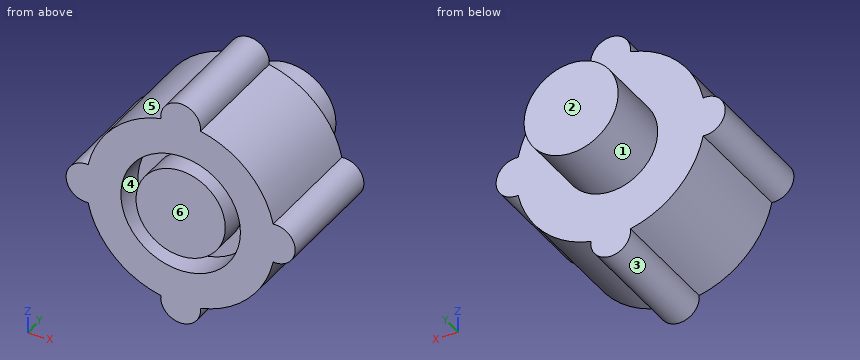
Autodesk Inventor part; units mm, degrees
ref_plane "YZ Plane" through (0, 0, 0) normal (1, 0, 0) x (0, 1, 0)
ref_plane "XZ Plane" through (0, 0, 0) normal (0, 1, 0) x (-1, 0, 0)
ref_plane "XY Plane" through (0, 0, 0) normal (0, 0, 1) x (1, 0, 0)
sketch "Sketch1" plane through (0, 0, 0) normal (0, 1, 0) x (-1, 0, 0)
  circle A0 centre (0, 0) radius 9.5
  dimension "d0" = 19
extrude "Extrusion1" add sketch "Sketch1" along normal blind 12
sketch "Sketch2" plane through (0, 12, 0) normal (0, 1, 0) x (1, 0, 0)
  circle A0 centre (0, 0) radius 4.7244
  dimension "d9" = 9.4488
extrude "Extrusion2" add sketch "Sketch2" along normal blind 6.9088
sketch "Sketch3" plane through (0, 0, 0) normal (0, -1, 0) x (1, 0, 0)
  circle A0 centre (0, 0) radius 4.48
  circle A1 centre (0, 0) radius 6
  dimension "d5" = 12
  dimension "d6" = 1.52
extrude "Extrusion3" cut sketch "Sketch3" against normal blind 3
sketch "Sketch4" plane through (0, 12, 0) normal (0, 1, 0) x (1, 0, 0)
  circle A0 centre (0, 0) radius 9.5
  circle A1 centre (-9.5, 0) radius 2
  line L0 (-15.7, 0) -> (13.7, 0)
  point P0 (-9.2895, 1.9889)
  point P1 (-9.2895, -1.9889)
  dimension "d10" = 4
extrude "Extrusion4" add sketch "Sketch4" against normal up to surface (12 mm away) contours A0 L0 A1 | A1 L0 A0 picked at (-10.0838, 0.5297) picked at (-10.0838, -0.5297)
pattern_circular "Circular Pattern1" count 4 over 360 about axis through (0, 0, 0) along (0, 1, 0) of "Extrusion4"
properties part number "Acople Resorte-Marcador"
Geometry: final body of the model. Coordinates: model frame, mm. Face numbers are marked on the shaded views. A direction names the side the tool comes from. Coordinates: 2 decimals unless noted, no trailing zeros. Order: outer loops, then holes, each group sorted by start corner. A loop starts at its lowest first (then second) coordinate and runs counter-clockwise, first axis right, second up.
(1) Draft query along X for the marked faces 3, 4, 5 and 6. Return one class per face: pulls with the +X half, pulls with the -X half, needs draft (parallel to the pull), parting line crosses it, or undercut.
(2) Material intervals for probe 1 along Z at (x, y) = (0, 2.3); probe 2 along Y at (x, z) = (2.5, -9); probe 3 along Z at (x, y) = (-5.5, 1.5), sorted ascending.
(3) Section query D-D (x = -5.25). Return the cut outline in (y, z).
(4) Section query A-A (y = 6.25). Return the cut outline in (x, z).
(5) Access query for the marked faces 1 and 2. Directions: +Z, -Z, +X, -X, +Y, -Y. A direction counts if a zero-diameter tool reaches every point of the face in a straight line with its end or side. Return the directions, or none.
(6) Section query C-C (x = 0). Return the cut outline in (y, z), plus the area to 3 significant figures.
(7) First-contact query: pin 1 (4 mm diameter, centred on y = 15, z = 5.5, fed in from -X); pin 2 (5 mm diameter, centred on x = 0.5, z = -8, fed in from +Y); pin 3 (3 mm diameter, centred on y = 7, z = 4, fed in from +X). Flat tips, straight axial feed; report the tip coordinate or a pass-through.
(8) Section query B-B (z = 0). Return the cut outline in (x, y).
Solution:
1. face 3: parting line crosses it
1. face 4: undercut
1. face 5: pulls with the -X half
1. face 6: needs draft
2. probe 1: z = -11.5 to -6, -4.48 to 4.48, 6 to 11.5
2. probe 2: y = 0 to 12
2. probe 3: z = -7.75 to -2.4, 2.4 to 7.75
3. outline: (0, -7.92) - (12, -7.92) - (12, 7.92) - (0, 7.92) - (0, 2.9) - (3, 2.9) - (3, -2.9) - (0, -2.9) - close
4. outline: (-9.29, -1.99) arc R9.5 ccw to (-1.99, -9.29) arc R2 ccw (long way) to (1.99, -9.29) arc R9.5 ccw to (9.29, -1.99) arc R2 ccw (long way) to (9.29, 1.99) arc R9.5 ccw to (1.99, 9.29) arc R2 ccw (long way) to (-1.99, 9.29) arc R9.5 ccw to (-9.29, 1.99) arc R2 ccw (long way) to start
5. face 1: +Y
5. face 2: +Z, -Z, +X, -X, +Y
6. outline: (0, -11.5) - (12, -11.5) - (12, -4.72) - (18.91, -4.72) - (18.91, 4.72) - (12, 4.72) - (12, 11.5) - (0, 11.5) - (0, 6) - (3, 6) - (3, 4.48) - (0, 4.48) - (0, -4.48) - (3, -4.48) - (3, -6) - (0, -6) - close
6. area: 332 mm2
7. pin 1: stops at x = -3.17
7. pin 2: stops at y = 12
7. pin 3: stops at x = 9.17
8. outline: (-11.5, 0) - (-6, 0) - (-6, 3) - (-4.48, 3) - (-4.48, 0) - (4.48, 0) - (4.48, 3) - (6, 3) - (6, 0) - (11.5, 0) - (11.5, 12) - (4.72, 12) - (4.72, 18.91) - (-4.72, 18.91) - (-4.72, 12) - (-11.5, 12) - close
